```python
from build123d import *

# Parameters (mm, degrees)
F1_DEPTH      = 700
F2_R          = 100
F3_DEPTH      = 400
F3_DEPTH_BACK = 310
F4_T          = -2.5


with BuildPart() as f1:
    # F0 (on Front) → F1 (new body)
    with BuildSketch(Plane.XZ):
        Polygon((270.7016063785, -167.6180982615), (124.1205126206, 332.3819017385), (-125.8794873794, 332.3819017385), (-229.2983936215, -167.6180982615), align=None)
    extrude(amount=-F1_DEPTH)

    # F2 (on Right) → F3 (cut, two sides)
    with BuildSketch(Plane.YZ) as f3_sk:
        with Locations((200, 332.3819017385)):
            Circle(F2_R)
        with Locations((500, 332.3819017385)):
            Circle(F2_R)
    extrude(amount=-F3_DEPTH, mode=Mode.SUBTRACT)
    extrude(f3_sk.sketch, amount=F3_DEPTH_BACK, mode=Mode.SUBTRACT)

    # F4
    f4_openings = [f1.faces().sort_by_distance(p)[0] for p in [
        (11.110009, 0, 54.604124),
        (203.411383, 350, 61.914311),
        (20.701606, 350, -167.618098),
        (-181.822412, 350, 61.914311),
        (11.110009, 700, 54.604124),
    ]]
    offset(amount=F4_T, openings=f4_openings)


solid = f1.part
```
Could you check a few things on this model? Use its own coordinates, in mm. A direction names the side the tool comes from. Round coordinates to 2 decimals unless told otherwise and drop trailing zeros. Loops run counter-clockwise (first coordinate to the right, second up) from the corner with the lowest first, then second, coordinate; pieces in that order, holes last.
Q1. For P1, Ø12, axis at x = 87.5, z = 288.5, coming from the -Y side; P2, Ø4, axis at x = -32, y = 143, coming from the +Z side; P3, Ø1, axis at x = -27.5, z = 242.5, coming from the +Y side, each with a flat end and sliding along its axis, tell me the tip position at first contact or that it passes through.
Q2. Thinking about a two-plate mould opening in Y: for faces 3 (the flat face through (1, 349, 329.882)), 4 (the flat face through (1, 651, 329.882)), which applies, pulls with the +Y half, pulls with the -Y half, needs draft (parallel to the pull), parting line crosses it, or undercut?
Q3. I want a section at C-C (y = 500). Write out the boundary of the cut face in (x, z).
Q4. I want a section at B-B (x = -43.5). Write out the boundary of the cut face in (y, z), and give its area (3 significant figures).
Q5. I want a section at A-A (z = 300). Write out the boundary of the cut face in (x, y), and give its area (3 significant figures).
Q6. I want a section at D-D (z = 272). Write out the boundary of the cut face in (x, y), and give its area (3 significant figures).
Q7. Please list where these lines run through material, in increasing order: L1, parallel to Y at x = 58, z = 305.5; L2, parallel to Y at x = 0, z = 266.5; L3, parallel to Z at x = -85.5, y = 317.5.
Q8. On a 3-axis mill with a long thin cutter (end or side, diameter ignored), from which of +Z, -Z, +X, -X, +Y, -Y can I reach the whole of each face in a straight line? I mean faces 1 (the flat face through (1, 48, 329.882)), 2 (the flat face through (124.75, 374.29, 330.24)). Say none if no direction works.
Answer below:
1. P1: stops at y = 104.76
1. P2: stops at z = 251.64
1. P3: stops at y = 550.17
2. face 3: undercut
2. face 4: needs draft
3. outline: (-147.08, 229.88) - (154.17, 229.88) - (153.44, 232.38) - (-146.56, 232.38) - close
4. outline: (0, 329.88) - (97.53, 329.88) arc R102.5 ccw to (302.47, 329.88) - (397.53, 329.88) arc R102.5 ccw to (602.47, 329.88) - (700, 329.88) - (700, 332.38) - (600, 332.38) arc R100 cw to (400, 332.38) - (300, 332.38) arc R100 cw to (100, 332.38) - (0, 332.38) - close
4. area: 2,320 mm2
5. outline: (-132.58, 102.75) - (133.61, 102.75) - (133.61, 105.39) - (-132.58, 105.39) - close; (-132.58, 294.61) - (133.61, 294.61) - (133.61, 297.25) - (-132.58, 297.25) - close; (-132.58, 402.75) - (133.61, 402.75) - (133.61, 405.39) - (-132.58, 405.39) - close; (-132.58, 594.61) - (133.61, 594.61) - (133.61, 597.25) - (-132.58, 597.25) - close
5. area: 2,810 mm2
6. outline: (-138.37, 117.17) - (141.82, 117.17) - (141.82, 120.29) - (-138.37, 120.29) - close; (-138.37, 279.71) - (141.82, 279.71) - (141.82, 282.83) - (-138.37, 282.83) - close; (-138.37, 417.17) - (141.82, 417.17) - (141.82, 420.29) - (-138.37, 420.29) - close; (-138.37, 579.71) - (141.82, 579.71) - (141.82, 582.83) - (-138.37, 582.83) - close
6. area: 3,490 mm2
7. L1: y = 101.09 to 103.68, 296.32 to 298.91, 401.09 to 403.68, 596.32 to 598.91
7. L2: y = 121.48 to 124.77, 275.23 to 278.52, 421.48 to 424.77, 575.23 to 578.52
7. L3: z = 329.88 to 332.38
8. face 1: -Z, +X, -X, -Y
8. face 2: +Z, +X, +Y, -Y
